Can you work these out from the model? Positions are in its coordinate system, mm. A direction names the side the tool comes from. Round coordinates to 2 decimals unless told otherwise and drop trailing zeros. Order: outer loops, then holes, each group sorted by start corner. A loop starts at its lowest first (then second) coordinate and runs counter-clockwise, first axis right, second up. Notation, with made-up numbers: M 65,53.5 L 97,53.5 A21 cw 97,82.5 Z; hole C 16,-20.75 d9. An arc over 180 degrees is marked long. Answer as a JSON object with one key per item and string values. Group by question number.
from build123d import *

# Parameters (mm, degrees)
SKETCH1_W                 = 63.5
SKETCH1_H                 = 63.5
SKETCH1_W_2               = 57.15
SKETCH1_H_2               = 57.15
EXTRUDE_THIN1_DEPTH       = 63.5
SKETCH2_W                 = 30
SKETCH2_H                 = 20
CUT_EXTRUDE1_DEPTH        = 64.5
SKETCH5_R                 = 7.5
CUT_EXTRUDE3_DEPTH        = 4.175
M3_CLEARANCE_HOLE1_D      = 3.6
M3_CLEARANCE_HOLE1_DEPTH  = 3.175
F_8_32_TAPPED_HOLE1_D     = 3.4544
F_8_32_TAPPED_HOLE1_DEPTH = 3.175
CUT_EXTRUDE4_REACH        = 65.5
SKETCH13_R                = 6
F_8_CLEARANCE_HOLE1_D     = 4.9149
F_8_CLEARANCE_HOLE1_DEPTH = 3.175


with BuildPart() as part:
    # Sketch1 → Extrude-Thin1 (new body)
    with BuildSketch(Plane.XY):
        Rectangle(SKETCH1_W, SKETCH1_H)
        Rectangle(SKETCH1_W_2, SKETCH1_H_2, mode=Mode.SUBTRACT)
    extrude(amount=EXTRUDE_THIN1_DEPTH)

    # Sketch2 → Cut-Extrude1 (cut, through all)
    with BuildSketch(Plane(origin=(31.75, 0, 0), x_dir=(0, 0, -1), z_dir=(1, 0, 0))):
        with Locations((-31.75, -31.75)):
            Rectangle(SKETCH2_W, SKETCH2_H)
    extrude(amount=-CUT_EXTRUDE1_DEPTH, mode=Mode.SUBTRACT)

    # Sketch5 → Cut-Extrude3 (cut, through all)
    with BuildSketch(Plane(origin=(28.575, 11.830115966, 29.988402314), x_dir=(0, 0, 1), z_dir=(-1, 0, 0))):
        with Locations((1.761597686, -13.580115966)):
            Circle(SKETCH5_R)
    extrude(amount=-CUT_EXTRUDE3_DEPTH, mode=Mode.SUBTRACT)

    # M3 Clearance Hole1
    with Locations(Plane(origin=(28.575, 11.830115966, 29.988402314), x_dir=(0, 0, 1), z_dir=(-1, 0, 0))):
        with Locations((-13.738402314, -6.580115966), (17.261597686, -6.580115966)):
            Hole(M3_CLEARANCE_HOLE1_D / 2, depth=M3_CLEARANCE_HOLE1_DEPTH)

    # #8-32 Tapped Hole1
    with Locations(Plane.ZY.offset(31.75)):
        with Locations((51.75, -1.75), (11.75, -1.75)):
            Hole(F_8_32_TAPPED_HOLE1_D / 2, depth=F_8_32_TAPPED_HOLE1_DEPTH)

    # Sketch13 → Cut-Extrude4 (cut, up to next)
    with BuildSketch(Plane.ZY.offset(31.75), mode=Mode.PRIVATE) as cut_extrude4_sk1:
        with Locations((31.75, -1.75)):
            Circle(SKETCH13_R)
    cut_extrude4_tool1 = extrude(cut_extrude4_sk1.sketch, amount=-CUT_EXTRUDE4_REACH, mode=Mode.PRIVATE) & part.part
    add(cut_extrude4_tool1.solids().sort_by_distance((-31.75, -1.75, 31.75))[0], mode=Mode.SUBTRACT)

    # #8 Clearance Hole1
    with Locations(Plane(origin=(0, -31.75, 0), x_dir=(-1, 0, 0), z_dir=(0, -1, 0))):
        with Locations((16, -8.75), (-16, -8.75), (-16, -54.75), (16, -54.75)):
            Hole(F_8_CLEARANCE_HOLE1_D / 2, depth=F_8_CLEARANCE_HOLE1_DEPTH)


solid = part.part
Item 1: On a 3-axis mill with a long thin cutter (end or side, diameter ignored), from which of +Z, -Z, +X, -X, +Y, -Y can I reach the whole of each face in a straight line? I mean faces 4 (the face through (-30.14, -1.231, 50.103)), 5 (the face through (17.321, -30.14, 52.678)), 6 (the face through (-30, -21.75, 32)), 7 (the face through (0, -28.575, 55)). Say none if no direction works.
Item 2: Suppose I cut it at B-B, the plane x = 16. Write out the boundary of the cut face in (y, z) (3 decimals), and give its area (3 significant figures).
Item 3: I'm going to push flat-ended pins straight in: pin 1 Ø3 at (x, z) = (10, 33) entering from -Y (3 decimals); pin 2 Ø1.6 at (x, z) = (30.5, 26.5) entering from -Y. Where does each tip first touch, or does it pass through?
Item 4: Suppose I cut it at C-C, the plane y = 14.5. Write out the boundary of the cut face in (x, z) (3 decimals), and give its area (3 significant figures).
Item 5: Suppose I cut it at D-D, the plane z = 31.75. Write out the boundary of the cut face in (x, y) (3 decimals).
Item 6: Suppose I cut it at A-A, the plane y = -25.5. Write out the boundary of the cut face in (x, z) (3 decimals), and give its area (3 significant figures).
Item 7: I need wall thicknesses on line 1 (Z direction, x = -16, y = -29); line 2 (Y direction, x = 30.2, z = 16.25); line 3 (Y direction, x = 11, z = 3.5) (3 decimals). Which ranges of each line are inside material? Lowest first, please.
Item 8: If we mould it in two halves opening along Z, with no side actions, what happens to faces 1 (the face through (-3, -30, 0)), 2 (the face through (-14.679, -30.14, 52.678)), 3 (the face through (0, 31.75, 31))? For each: +Z half, -Z half, draft (parallel to the pull), parting line (faces both ways), or undercut.
Computed:
{
 "1": {"face 4": "-X", "face 5": "-Y", "face 6": "+X, -X, -Y", "face 7": "+Z, -Z"},
 "2": {"outline": "M -31.75,0 L -28.575,0 L -28.575,6.293 L -31.75,6.293 Z; M -31.75,11.207 L -28.575,11.207 L -28.575,16.75 L -31.75,16.75 Z; M -31.75,46.75 L -28.575,46.75 L -28.575,52.293 L -31.75,52.293 Z; M -31.75,57.207 L -28.575,57.207 L -28.575,63.5 L -31.75,63.5 Z; M 28.575,0 L 31.75,0 L 31.75,63.5 L 28.575,63.5 Z", "area": "277 mm^2"},
 "3": {"pin 1": "stops at y = 28.575", "pin 2": "stops at y = -21.75"},
 "4": {"outline": "M -31.75,0 L -28.575,0 L -28.575,63.5 L -31.75,63.5 Z; M 28.575,0 L 31.75,0 L 31.75,63.5 L 28.575,63.5 Z", "area": "403 mm^2"},
 "5": {"outline": "M -31.75,-21.75 L -28.575,-21.75 L -28.575,-7.75 L -31.75,-7.75 Z; M -31.75,4.25 L -28.575,4.25 L -28.575,28.575 L 28.575,28.575 L 28.575,5.75 L 31.75,5.75 L 31.75,31.75 L -31.75,31.75 Z; M 28.575,-21.75 L 31.75,-21.75 L 31.75,-9.25 L 28.575,-9.25 Z"},
 "6": {"outline": "M -31.75,0 L -28.575,0 L -28.575,16.75 L -31.75,16.75 Z; M -31.75,46.75 L -28.575,46.75 L -28.575,63.5 L -31.75,63.5 Z; M 28.575,0 L 31.75,0 L 31.75,16.75 L 28.575,16.75 Z; M 28.575,46.75 L 31.75,46.75 L 31.75,63.5 L 28.575,63.5 Z", "area": "213 mm^2"},
 "7": {"line 1": "z = 0 to 6.29, 11.21 to 16.75, 46.75 to 52.29, 57.21 to 63.5", "line 2": "y = -31.75 to 3.45, 7.05 to 31.75", "line 3": "y = -31.75 to -28.575, 28.575 to 31.75"},
 "8": {"face 1": "-Z half", "face 2": "undercut", "face 3": "draft"}
}
